Geometry check sheet. Reference: the model listing, model coordinates, mm. A direction names the side the tool comes from. Coordinates: 2 decimals unless noted, no trailing zeros. Write each loop counter-clockwise with the first axis right and the second up, starting at its lowest first coordinate (ties: lowest second). Pieces come first, ordered by that corner, then holes. Notation, with made-up numbers: (71, 0.5) -> (85, 0.5) arc R20 cw to (85, 24.5) -> close; hole circle Ø4 at (71, 14). An arc over 180 degrees is marked (long way). Use a Markdown table: item, result.
```python
from build123d import *

# Parameters (mm, degrees)
SKETCH1_W               = 304.8
SKETCH1_H               = 127
BOSS_EXTRUDE1_DEPTH     = 101.6
SHELL1_T                = 6.35
CUT_EXTRUDE1_DEPTH      = 223.88409544
CUT_EXTRUDE1_DEPTH_BACK = 223.88409544
SKETCH2_W               = 254
SKETCH2_H               = 19.05


with BuildPart() as part:
    # Sketch1 → Boss-Extrude1 (new body)
    with BuildSketch(Plane(origin=(0, 0, 0), x_dir=(1, 0, 0), z_dir=(0, 1, 0))):
        Rectangle(SKETCH1_W, SKETCH1_H)
    extrude(amount=BOSS_EXTRUDE1_DEPTH)

    # Shell1 (no face opened: a closed hollow body)
    add(offset(amount=-SHELL1_T, mode=Mode.PRIVATE), mode=Mode.SUBTRACT)

    # Sketch2 → Cut-Extrude1 (cut, two sides: drawn at the far end of the back side and taken through both)
    with BuildSketch(Plane.XY.offset(63.5).offset(-CUT_EXTRUDE1_DEPTH_BACK)):
        with Locations((0, 12.7)):
            Rectangle(SKETCH2_W, SKETCH2_H)
    extrude(amount=CUT_EXTRUDE1_DEPTH + CUT_EXTRUDE1_DEPTH_BACK, mode=Mode.SUBTRACT)


solid = part.part
```
Item 1: Section check A-A on x = 19.5. Record the boundary of the cut face in (y, z) (3 decimals), then the cut area to 3 significant figures.
Answer block:
| item | result |
|---|---|
| outline | (0, -63.5) -> (3.175, -63.5) -> (3.175, 63.5) -> (0, 63.5) -> close; (22.225, -63.5) -> (101.6, -63.5) -> (101.6, 63.5) -> (22.225, 63.5) -> (22.225, 57.15) -> (95.25, 57.15) -> (95.25, -57.15) -> (22.225, -57.15) -> close |
| area | 2,140 mm^2 |
Item 2: Section check D-D on y = 90. Record the boundary of the cut face in (x, z), then the cut area to 3 significant figures.
Answer block:
| item | result |
|---|---|
| outline | (-152.4, -63.5) -> (152.4, -63.5) -> (152.4, 63.5) -> (-152.4, 63.5) -> close; hole (-146.05, -57.15) -> (146.05, -57.15) -> (146.05, 57.15) -> (-146.05, 57.15) -> close |
| area | 5,320 mm^2 |
Item 3: Section check B-B on y = 11.5. Record the boundary of the cut face in (x, z), then the cut area to 3 significant figures.
Answer block:
| item | result |
|---|---|
| outline | (-152.4, -63.5) -> (-127, -63.5) -> (-127, -57.15) -> (-146.05, -57.15) -> (-146.05, 57.15) -> (-127, 57.15) -> (-127, 63.5) -> (-152.4, 63.5) -> close; (127, -63.5) -> (152.4, -63.5) -> (152.4, 63.5) -> (127, 63.5) -> (127, 57.15) -> (146.05, 57.15) -> (146.05, -57.15) -> (127, -57.15) -> close |
| area | 2,100 mm^2 |
Item 4: Section check C-C on z = -52. Record the boundary of the cut face in (x, y) (3 decimals), then the cut area to 3 significant figures.
Answer block:
| item | result |
|---|---|
| outline | (-152.4, 0) -> (152.4, 0) -> (152.4, 101.6) -> (-152.4, 101.6) -> close; hole (-146.05, 6.35) -> (-127, 6.35) -> (-127, 3.175) -> (127, 3.175) -> (127, 6.35) -> (146.05, 6.35) -> (146.05, 95.25) -> (-146.05, 95.25) -> close |
| area | 4,190 mm^2 |
Item 5: Thickness scan on L1, parallel to X at y = 78.5, z = -32.5; L2, parallel to Y at x = -121, z = -34 (3 decimals); L3, parallel to Z at x = 34.5, y = 94. Record the ranges inside material, lowest first. Write a range as [from, to].
Answer block:
| item | result |
|---|---|
| L1 | x = [-152.4, -146.05], [146.05, 152.4] |
| L2 | y = [0, 3.175], [95.25, 101.6] |
| L3 | z = [-63.5, -57.15], [57.15, 63.5] |
Item 6: Mould release check, pull along Z, two halves, no side actions. Record for faces 4 (the flat face through (136, 6.35, -1)), 5 (the flat face through (-2, 61, -63.5)), 6 (the flat face through (-127, 6, -14)), 7 (the flat face through (146.05, 50, 1)): +Z half, -Z half, draft (parallel to the pull), parting line (faces both ways), or undercut.
Answer block:
| item | result |
|---|---|
| face 4 | undercut |
| face 5 | -Z half |
| face 6 | draft |
| face 7 | undercut |
Item 7: Tool access check on faces 1 (the flat face through (-2, 22.225, 60)), 2 (the flat face through (-2, 61, 63.5)), 3 (the flat face through (-2, 60, 57.15)). Record the directions out of +Z, -Z, +X, -X, +Y, -Y that give a thin tool (end or side, any length) a straight path to the whole face; none if there is none.
Answer block:
| item | result |
|---|---|
| face 1 | +Z, -Z |
| face 2 | +Z, +X, -X, +Y, -Y |
| face 3 | none |
